Model file for the job. Use its own axes, mm. A direction names the side the tool comes from. Coordinates: 2 decimals unless noted, no trailing zeros. Write each loop counter-clockwise with the first axis right and the second up, starting at its lowest first coordinate (ties: lowest second). Pieces come first, ordered by that corner, then holes. Notation, with made-up numbers: M 22,-11.5 L 73,-11.5 A24 ccw 73,-1.5 Z; hole C 35,-9 d7. An arc over 180 degrees is marked long. Answer in a Markdown table with one row per item. Add a question column.
Autodesk Fusion 360 part; units mm, degrees
sketch "Front-OuterDimensionsAndHoles" plane through (0, 0, 0) normal (0, 1, 0) x (1, 0, 0) in component "1006351A-GASKET"
  line L0 (-137.0277, -51.6717) -> (147.7462, -51.6717) construction
  line L1 (-113.1932, -37.4477) -> (126.9355, -37.4477) construction
  line L2 (-111.6736, 46.3723) -> (88.9542, 46.3723) construction
  line L3 (-83.38, 4.4623) -> (113.9408, 4.4623) construction
  line L4 (77.012, -30.3357) -> (138.7437, -30.3357) construction
  line L5 (77.3795, 43.3243) -> (102.1824, 43.3243) construction
  line L6 (-79.2352, -152.4901) -> (-79.2352, 67.7682) construction
  line L7 (80.7848, -152.4901) -> (80.7848, 99.4049) construction
  line L8 (-16.2432, -127.3246) -> (-16.2432, -37.4477) construction
  line L9 (-61.4552, -139.7875) -> (-61.4552, -23.5467) construction
  line L10 (-4.5592, -114.8617) -> (-4.5592, -39.3651) construction
  line L11 (0.7748, -102.6384) -> (0.7748, 79.7518) construction
  line L12 (6.1088, -89.6961) -> (6.1088, 17.4372) construction
  line L13 (122.5447, -1.8877) -> (-114.7303, -1.8877) construction
  line L14 (151.0657, 56.0243) -> (-121.6808, 56.0243) construction
  line L15 (-84.366, -162.1054) -> (-84.366, 89.1529) construction
  line L16 (84.8488, -151.7017) -> (84.8488, 106.4269) construction
  line L17 (17.7928, -77.6983) -> (17.7928, -42.3651) construction
  line L18 (63.0048, -65.3317) -> (63.0048, -43.9355) construction
  line L19 (-137.1695, 60.5963) -> (174.7441, 60.5963) construction
  line L20 (-87.8994, -47.0997) -> (156.6849, -47.0997) construction
  line L21 (70.6248, 70.8097) -> (70.6248, -45.2683) construction
  line L22 (16.2688, 71.2679) -> (16.2688, -42.3651) construction
  line L23 (-15.786, 70.5042) -> (-15.786, -42.9773) construction
  line L24 (-70.142, 108.0768) -> (-70.142, -44.9628) construction
  line L25 (-10.9092, 93.2616) -> (-10.9092, -44.6574) construction
  line L26 (73.9383, 85.014) -> (73.9383, -42.8245) construction
  line L27 (-101.4005, 49.5796) -> (76.5348, 49.5796) construction
  line L28 (-100.0259, -41.454) -> (76.8403, -41.454) construction
  line L29 (-78.8288, -51.9257) -> (79.3116, -51.9257)
  line L30 (84.8488, -46.3885) -> (84.8488, 54.8051)
  line L31 (79.3116, 60.3423) -> (-78.8288, 60.3423)
  line L32 (-84.366, 54.8051) -> (-84.366, -46.3885)
  line L33 (-66.967, -37.7017) -> (-18.961, -37.7017)
  line L34 (-15.786, -34.5267) -> (-15.786, 42.9433)
  line L35 (-18.961, 46.1183) -> (-66.967, 46.1183)
  line L36 (-70.142, 42.9433) -> (-70.142, -34.5267)
  line L37 (19.4438, -37.7017) -> (67.4498, -37.7017)
  line L38 (70.6248, -34.5267) -> (70.6248, 42.9433)
  line L39 (67.4498, 46.1183) -> (19.4438, 46.1183)
  line L40 (16.2688, 42.9433) -> (16.2688, -34.5267)
  arc A0 (-84.366, -46.3885) -> (-78.8288, -51.9257) centre (-78.8288, -46.3885) ccw
  arc A1 (-78.8288, 60.3423) -> (-84.366, 54.8051) centre (-78.8288, 54.8051) ccw
  arc A2 (84.8488, 54.8051) -> (79.3116, 60.3423) centre (79.3116, 54.8051) ccw
  arc A3 (-70.142, -34.5267) -> (-66.967, -37.7017) centre (-66.967, -34.5267) ccw
  arc A4 (-18.961, -37.7017) -> (-15.786, -34.5267) centre (-18.961, -34.5267) ccw
  arc A5 (-15.786, 42.9433) -> (-18.961, 46.1183) centre (-18.961, 42.9433) ccw
  arc A6 (-66.967, 46.1183) -> (-70.142, 42.9433) centre (-66.967, 42.9433) ccw
  arc A7 (67.4498, -37.7017) -> (70.6248, -34.5267) centre (67.4498, -34.5267) ccw
  arc A8 (70.6248, 42.9433) -> (67.4498, 46.1183) centre (67.4498, 42.9433) ccw
  arc A9 (19.4438, 46.1183) -> (16.2688, 42.9433) centre (19.4438, 42.9433) ccw
  arc A10 (16.2688, -34.5267) -> (19.4438, -37.7017) centre (19.4438, -34.5267) ccw
  arc A11 (79.3116, -51.9257) -> (84.8488, -46.3885) centre (79.3116, -46.3885) ccw
  line L41 (-100.3246, -43.4352) -> (86.6573, -43.4352) construction
  line L42 (-99.9078, -39.4728) -> (77.154, -39.4728) construction
  line L43 (-94.8446, 47.5984) -> (76.1721, 47.5984) construction
  line L44 (-94.4522, 51.5608) -> (76.1721, 51.5608) construction
  line L45 (-73.1392, 86.7279) -> (-73.1392, -45.4577) construction
  line L46 (-8.928, 72.5566) -> (-8.928, -44.6167) construction
  line L47 (-12.8904, 72.2199) -> (-12.8904, -44.6167) construction
  line L48 (-75.1204, 70.9572) -> (-75.1204, -44.6167) construction
  line L49 (-71.158, 71.0414) -> (-71.158, -44.3641) construction
  line L50 (-66.967, 51.5608) -> (-17.0814, 51.5608)
  line L51 (-8.928, 43.4074) -> (-8.928, -35.2818)
  line L52 (-17.0814, -43.4352) -> (-66.967, -43.4352)
  line L53 (-75.1204, -35.2818) -> (-75.1204, 43.4074)
  line L54 (-66.205, 47.5984) -> (-17.8434, 47.5984)
  line L55 (-12.8904, 42.6454) -> (-12.8904, -34.5198)
  line L56 (-17.8434, -39.4728) -> (-66.205, -39.4728)
  line L57 (-71.158, -34.5198) -> (-71.158, 42.6454)
  arc A12 (-75.1204, -35.2818) -> (-66.967, -43.4352) centre (-66.967, -35.2818) ccw
  arc A13 (-17.0814, -43.4352) -> (-8.928, -35.2818) centre (-17.0814, -35.2818) ccw
  arc A14 (-8.928, 43.4074) -> (-17.0814, 51.5608) centre (-17.0814, 43.4074) ccw
  arc A15 (-66.967, 51.5608) -> (-75.1204, 43.4074) centre (-66.967, 43.4074) ccw
  arc A16 (-71.158, -34.5198) -> (-66.205, -39.4728) centre (-66.205, -34.5198) ccw
  arc A17 (-66.205, 47.5984) -> (-71.158, 42.6454) centre (-66.205, 42.6454) ccw
  arc A18 (-12.8904, 42.6454) -> (-17.8434, 47.5984) centre (-17.8434, 42.6454) ccw
  arc A19 (-17.8434, -39.4728) -> (-12.8904, -34.5198) centre (-17.8434, -34.5198) ccw
  line L58 (18.631, -43.4352) -> (68.5166, -43.4352)
  arc A20 (68.5166, -43.4352) -> (76.67, -35.2818) centre (68.5166, -35.2818) ccw
  line L59 (76.67, -35.2818) -> (76.67, 43.4074)
  arc A21 (76.67, 43.4074) -> (68.5166, 51.5608) centre (68.5166, 43.4074) ccw
  line L60 (68.5166, 51.5608) -> (18.631, 51.5608)
  arc A22 (18.631, 51.5608) -> (10.4776, 43.4074) centre (18.631, 43.4074) ccw
  line L61 (10.4776, 43.4074) -> (10.4776, -35.2818)
  arc A23 (10.4776, -35.2818) -> (18.631, -43.4352) centre (18.631, -35.2818) ccw
  line L62 (19.393, -39.4728) -> (67.7546, -39.4728)
  arc A24 (67.7546, -39.4728) -> (72.7076, -34.5198) centre (67.7546, -34.5198) ccw
  line L63 (72.7076, -34.5198) -> (72.7076, 42.6454)
  arc A25 (72.7076, 42.6454) -> (67.7546, 47.5984) centre (67.7546, 42.6454) ccw
  line L64 (67.7546, 47.5984) -> (19.393, 47.5984)
  arc A26 (19.393, 47.5984) -> (14.44, 42.6454) centre (19.393, 42.6454) ccw
  line L65 (14.44, 42.6454) -> (14.44, -34.5198)
  line L66 (101.4573, -39.4728) -> (-75.6045, -39.4728) construction
  arc A27 (14.44, -34.5198) -> (19.393, -39.4728) centre (19.393, -34.5198) ccw
  point P0 (-79.2352, -47.0997)
  point P1 (-4.5592, -47.0997)
  point P2 (6.1088, -47.0997)
  point P3 (80.7848, -47.0997)
  point P4 (80.7848, 4.4623)
  point P5 (6.1088, 4.4623)
  point P6 (-79.2352, 4.4623)
  point P7 (-4.5592, 4.4623)
  point P8 (80.7848, 56.0243)
  point P9 (6.1088, 56.0243)
  point P10 (-4.5592, 56.0243)
  point P11 (-79.2352, 56.0243)
  point P12 (80.7848, -30.3357)
  point P13 (80.7848, 43.3243)
  point P14 (63.0048, -47.0997)
  point P15 (17.7928, -47.0997)
  point P16 (17.7928, 56.0243)
  point P17 (63.0048, 56.0243)
  point P18 (0.7748, -1.8877)
  point P19 (-16.2432, -47.0997)
  point P20 (-61.4552, -47.0997)
  point P21 (-79.2352, -30.3357)
  point P22 (-79.2352, 43.3243)
  point P23 (-61.4552, 56.0243)
  point P24 (-16.2432, 56.0243)
  dimension "d1" = 169.2148
  dimension "d2" = 4.064
  dimension "d3" = 160.02
  dimension "d4" = 142.24
  dimension "d5" = 97.028
  dimension "d6" = 85.344
  dimension "d7" = 80.01
  dimension "d8" = 74.676
  dimension "d9" = 17.78
  dimension "d10" = 62.992
  dimension "d12" = 112.268
  dimension "d13" = 103.124
  dimension "d14" = 51.562
  dimension "d16" = 57.912
  dimension "d17" = 86.36
  dimension "d18" = 12.7
  dimension "d19" = 14.224
  dimension "d20" = 4.572
  dimension "d21" = 14.224
  dimension "d22" = 14.224
  dimension "d23" = 54.356
  dimension "d24" = 54.356
  dimension "d25" = 91.0336
  dimension "d26" = 14.224
  dimension "d27" = 5.5372
  dimension "d28" = 5.5372
  dimension "d29" = 5.5372
  dimension "d30" = 3.175
  dimension "d31" = 3.175
  dimension "d32" = 3.175
  dimension "d33" = 3.175
  dimension "d34" = 3.175
  dimension "d35" = 3.175
  dimension "d36" = 3.175
  dimension "d37" = 3.175
  dimension "d40" = 5.5372
  dimension "d49" = 1.9812
  dimension "d50" = 1.9812
  dimension "d51" = 1.9812
  dimension "d52" = 1.9812
  dimension "d53" = 91.694
  dimension "d54" = 62.23
  dimension "d55" = 1.9812
  dimension "d56" = 1.9812
  dimension "d57" = 1.9812
  dimension "d58" = 1.9812
  dimension "d59" = 8.1534
  dimension "d60" = 8.1534
  dimension "d61" = 8.1534
  dimension "d62" = 8.1534
  dimension "d63" = 4.953
  dimension "d64" = 4.953
  dimension "d65" = 4.953
  dimension "d66" = 4.953
extrude "Extrude1" add sketch "Front-OuterDimensionsAndHoles" along normal blind 3.2004 contours L29 L30 L31 L32 A0 A1 A2 A11 | L50 L51 L52 L53 A12 A13 A14 A15 | L54 L55 L56 L57 A16 A17 A18 A19 | L58 A20 L59 A21 L60 A22 L61 A23 | L62 A24 L63 A25 L64 A26 L65 A27 in component "1006351A-GASKET"
hole "Hole1" at (80.7848, 0, 47.0997) at (6.1088, 0, 47.0997) at (-4.5592, 0, 47.0997) at (-79.2352, 0, 47.0997) at (-79.2352, 0, -56.0243) at (6.1088, 0, -56.0243) at (-4.5592, 0, -56.0243) at (80.7848, 0, -56.0243) at (80.7848, 0, -4.4623) at (6.1088, 0, -4.4623) at (-4.5592, 0, -4.4623) at (-79.2352, 0, -4.4623) direction (0, 1, 0) diameter 4.572 end through all in component "1006351A-GASKET"
hole "Hole2" at (-61.4552, 0, 47.0997) at (-16.2432, 0, 47.0997) at (17.7928, 0, 47.0997) at (63.0048, 0, 47.0997) at (80.7848, 0, 30.3357) at (80.7848, 0, -43.3243) at (63.0048, 0, -56.0243) at (0.7748, 0, 1.8877) at (-16.2432, 0, -56.0243) at (17.7928, 0, -56.0243) at (-61.4552, 0, -56.0243) at (-79.2352, 0, -43.3243) at (-79.2352, 0, 30.3357) direction (0, 1, 0) diameter 3.3782 end through all countersink diameter 5.842 countersink angle 82 in component "1006351A-GASKET"
extrude "Extrude2" cut sketch "Front-OuterDimensionsAndHoles" along normal blind 0.6604 contours L50 L51 L52 L53 A12 A13 A14 A15 | L58 A20 L59 A21 L60 A22 L61 A23 in component "1006351A-GASKET"
component "1006351A-GASKET" placed x (1, 0, 0) y (0, 1, 0) z (0, 0, 1) at (0, 0, 0)
equation "d49 = ( 0.156 / 2 ) * 1 in"
equation "d50 = ( 0.156 / 2 ) * 1 in"
equation "d51 = ( 0.156 / 2 ) * 1 in"
equation "d52 = ( 0.156 / 2 ) * 1 in"
1) Two-plate mould, pull along X, no slides. Class faces 3 (the face through (-1, 3.2, -5)), 4 (the face through (-82.7, 1.58, 50.35)), 5 (the face through (71.218, 0.326, -46.186)), 6 (the face through (-72.795, 0.326, -49.109)): released by +X, released by -X, zero draft, split by the parting line, or undercut.
2) Slice it at A-A (z = 9.5). Give the cut face in (x, y), then the cut area to 3 significant figures.
3) Which spindle directions (+Z, -Z, +X, -X, +Y, -Y) get a long thin tool onto all of the face, cutting with end or side? Do faces 1 (the face through (69.67, 1.578, -45.213)), 2 (the face through (74.345, 0.326, 40.983)). Say none if no direction does.
4) Drill centre lines: probe 1 along X at (y, z) = (2.35, 19); probe 2 along Z at (x, y) = (-62, 1.3); probe 3 along X at (y, z) = (0.9, -42). Where is each one in solid material? Low to high.
5) Slice it at C-C (y = 2.6). Count the separate pieces of the cut face and the enclosed holes in it, then the cut area to 3 significant figures.
6) Flat gauge pins, fed straight in: pin 1 Ø3.5 at (x, z) = (6.11, 47.1) entering from -Y; pin 2 Ø5.5 at (x, z) = (-61.46, 47.1) entering from -Y. Where does each tip first touch, or does it go through?
7) Slice it at B-B (x = -32). Give the cut face in (y, z), then the cut area to 3 significant figures.
Ans:
| question | item | result |
|---|---|---|
| 1 | face 3 | zero draft |
| 1 | face 4 | released by -X |
| 1 | face 5 | undercut |
| 1 | face 6 | undercut |
| 2 | outline | M -84.37,0 L -75.12,0 L -75.12,0.66 L -71.16,0.66 L -71.16,0 L -70.14,0 L -70.14,3.2 L -84.37,3.2 Z; M -15.79,0 L -12.89,0 L -12.89,0.66 L -8.93,0.66 L -8.93,0 L 10.48,0 L 10.48,0.66 L 14.44,0.66 L 14.44,0 L 16.27,0 L 16.27,3.2 L -15.79,3.2 Z; M 70.62,0 L 72.71,0 L 72.71,0.66 L 76.67,0.66 L 76.67,0 L 84.85,0 L 84.85,3.2 L 70.62,3.2 Z |
| 2 | area | 183 mm2 |
| 3 | face 1 | +Y, -Y |
| 3 | face 2 | -Y |
| 4 | probe 1 | x = -84.37 to -70.14, -15.79 to 16.27, 70.62 to 84.85 |
| 4 | probe 2 | z = -60.34 to -57.73, -54.32 to -46.12, 37.7 to 45.39, 48.81 to 51.93 |
| 4 | probe 3 | x = -84.37 to -80.91, -77.56 to -70.14, -15.79 to 16.27, 70.62 to 79.11, 82.46 to 84.85 |
| 5 | separate pieces | 1 |
| 5 | enclosed holes | 27 |
| 5 | area | 9,560 mm2 |
| 6 | pin 1 | passes through |
| 6 | pin 2 | stops at y = 0.19 |
| 7 | outline | M 0,-60.34 L 3.2,-60.34 L 3.2,-46.12 L 0,-46.12 L 0,-47.6 L 0.66,-47.6 L 0.66,-51.56 L 0,-51.56 Z; M 0,37.7 L 3.2,37.7 L 3.2,51.93 L 0,51.93 L 0,43.44 L 0.66,43.44 L 0.66,39.47 L 0,39.47 Z |
| 7 | area | 85.8 mm2 |
